The listing builds one solid part. Answer for the finished solid, in the listing's coordinates (mm). Face numbers are marked on the shaded views. A direction names the side the tool comes from. Coordinates: 2 decimals unless noted, no trailing zeros. Loops run counter-clockwise (first coordinate to the right, second up) from the corner with the lowest first, then second, coordinate; pieces in that order, holes last. Notation, with made-up numbers: (-6, 12.5) - (14, 12.5) arc R25 ccw to (14, 24.5) - close; hole circle Ø8 at (-38.75, 32). An arc over 180 degrees is marked (long way). Put each result on its own line as item: value.
```python
from build123d import *

# Parameters (mm, degrees)
SKETCH1_W               = 120
SKETCH1_H               = 31.25
BOSS_EXTRUDE1_DEPTH     = 7
SKETCH2_W               = 120
SKETCH2_H               = 4
SKETCH2_H_2             = 1
BOSS_EXTRUDE2_DEPTH     = 8
CUT_EXTRUDE1_DEPTH      = 125.260059955
CUT_EXTRUDE1_DEPTH_BACK = 125.260059955
SKETCH3_W               = 102
SKETCH3_H               = 8
SKETCH3_H_2             = 3.5
CUT_EXTRUDE3_REACH      = 126.906
SKETCH6_W               = 5
SKETCH6_H               = 1
SKETCH4_W               = 3
SKETCH4_H               = 8.090611825
SKETCH4_H_2             = 10.659388175
CUT_EXTRUDE4_DEPTH      = 5
SKETCH5_W               = 2.75
SKETCH5_H               = 7.59
SKETCH5_H_2             = 11.2
BOSS_EXTRUDE3_DEPTH     = 5
SKETCH7_R               = 3.1
CUT_EXTRUDE5_DEPTH      = 4
CUT_EXTRUDE6_START      = -1
SKETCH8_R               = 3.1
CUT_EXTRUDE6_DEPTH      = 1
CHAMFER1_SIZE           = 1


with BuildPart() as part:
    # Sketch1 → Boss-Extrude1 (new body)
    with BuildSketch(Plane.XY):
        with Locations((60, 15.625)):
            Rectangle(SKETCH1_W, SKETCH1_H)
    extrude(amount=BOSS_EXTRUDE1_DEPTH)

    # Sketch2 → Boss-Extrude2 (add)
    with BuildSketch(Plane.XY.offset(7)):
        with Locations((60, 25.6)):
            Rectangle(SKETCH2_W, SKETCH2_H)
        with Locations((60, 0.5)):
            Rectangle(SKETCH2_W, SKETCH2_H_2)
    extrude(amount=BOSS_EXTRUDE2_DEPTH)

    # Sketch3 → Cut-Extrude1 (cut, two sides: drawn at the far end of the back side and taken through both)
    with BuildSketch(Plane.XY.offset(7).offset(-CUT_EXTRUDE1_DEPTH_BACK)):
        with Locations((61, 11.1)):
            Rectangle(SKETCH3_W, SKETCH3_H)
        with Locations((61, 21.85)):
            Rectangle(SKETCH3_W, SKETCH3_H_2)
    extrude(amount=CUT_EXTRUDE1_DEPTH + CUT_EXTRUDE1_DEPTH_BACK, mode=Mode.SUBTRACT)

    # Sketch6 → Cut-Extrude3 (cut, up to next)
    with BuildSketch(Plane.ZY, mode=Mode.PRIVATE) as cut_extrude3_sk1:
        with Locations((12.5, 0.5)):
            Rectangle(SKETCH6_W, SKETCH6_H)
    cut_extrude3_tool1 = extrude(cut_extrude3_sk1.sketch, amount=-CUT_EXTRUDE3_REACH, mode=Mode.PRIVATE) & part.part
    add(cut_extrude3_tool1.solids().sort_by_distance((0, 0.5, 12.5))[0], mode=Mode.SUBTRACT)

    # Sketch4 → Cut-Extrude4 (cut)
    with BuildSketch(Plane.ZY):
        with Locations((3.5, 24.204694088)):
            Rectangle(SKETCH4_W, SKETCH4_H)
        with Locations((3.5, 8.829694088)):
            Rectangle(SKETCH4_W, SKETCH4_H_2)
    extrude(amount=-CUT_EXTRUDE4_DEPTH, mode=Mode.SUBTRACT)

    # Sketch5 → Boss-Extrude3 (add)
    with BuildSketch(Plane(origin=(120, 0, 0), x_dir=(0, 0, -1), z_dir=(1, 0, 0))):
        with Locations((-3.5, 24.205)):
            Rectangle(SKETCH5_W, SKETCH5_H)
        with Locations((-3.5, 9.35)):
            Rectangle(SKETCH5_W, SKETCH5_H_2)
    extrude(amount=BOSS_EXTRUDE3_DEPTH)

    # Sketch7 → Cut-Extrude5 (cut)
    with BuildSketch(Plane.XY.offset(7)):
        with Locations((116, 15.1)):
            Circle(SKETCH7_R)
    extrude(amount=-CUT_EXTRUDE5_DEPTH, mode=Mode.SUBTRACT)

    # Sketch8 → Cut-Extrude6 (cut)
    with BuildSketch(Plane(origin=(0, 0, 0), x_dir=(-1, 0, 0), z_dir=(0, 0, -1)).offset(CUT_EXTRUDE6_START)):
        with Locations(Location((-116, 15.1, 0), (0, 0, 180))):
            Circle(SKETCH8_R)
    extrude(amount=CUT_EXTRUDE6_DEPTH, mode=Mode.SUBTRACT)

    # Chamfer1
    chamfer1_edges = [part.edges().sort_by_distance(p)[0] for p in [
        (112.9, 15.1, 1),
    ]]
    chamfer(chamfer1_edges, length=CHAMFER1_SIZE - 0.0001)  # a hair under: the kernel refuses the full size


solid = part.part
```
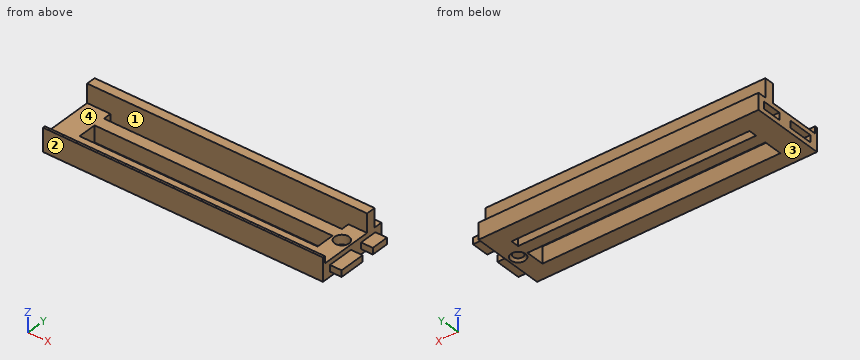
1) The part is cut by section B-B (z = 8.25). Give the vertices of the cut face in (x, y), and give its area (3 significant figures).
Found:
outline: (0, 0) - (120, 0) - (120, 1) - (0, 1) - close; (0, 23.6) - (120, 23.6) - (120, 27.6) - (0, 27.6) - close
area: 600 mm^2
2) Each of these flat-tipped pins is pushed along its axis until it touches: pin 1 (11.5 mm diameter, centred on x = 70, y = 8, fed in from +Z); pin 2 (3 mm diameter, centred on x = 38.5, y = 13, fed in from -Z); pin 3 (0.8 mm diameter, centred on x = 40.5, y = 0.5, fed in from +Z); pin 4 (1.4 mm diameter, centred on x = 123, z = 3, fed in from +Y). Where does it stop, or does it pass through?
Found:
pin 1: stops at z = 7
pin 2: passes through
pin 3: stops at z = 10
pin 4: stops at y = 28
3) The part is cut by section D-D (y = 5). Give the vertices of the cut face in (x, z) (3 decimals).
Found:
outline: (0, 0) - (120, 0) - (120, 2.125) - (125, 2.125) - (125, 4.875) - (120, 4.875) - (120, 7) - (0, 7) - (0, 5) - (5, 5) - (5, 2) - (0, 2) - close
4) For a pull along X with two mould halves and no side action, classify the marked faces 1 and 2 as pulls with the +X half, pulls with the -X half, needs draft (parallel to the pull), parting line crosses it, or undercut.
Found:
face 1: undercut
face 2: needs draft
5) For the marked faces 3 and 4, determine the directions among +Z, -Z, +X, -X, +Y, -Y from which every point of the face is accessible in a straight line to the end or side of a thin tool.
Found:
face 3: -Z, +X, -X, +Y, -Y
face 4: +Z, +X, -X
6) Straight lines are drawn through the part: L1, parallel to Y at x = 97.5, z = 4.75; L2, parallel to Y at x = 61.5, z = 9.25; L3, parallel to Y at x = 53, z = 14.75. For each, find the intervals that lie inside material, in ascending order. Write a range as [from, to].
Found:
L1: y = [0, 7.1], [15.1, 20.1], [23.6, 31.25]
L2: y = [0, 1], [23.6, 27.6]
L3: y = [23.6, 27.6]
7) The part is cut by section A-A (x = 31.5). Give the vertices of the cut face in (y, z), and give its area (3 significant figures).
Found:
outline: (0, 0) - (7.1, 0) - (7.1, 7) - (1, 7) - (1, 10) - (0, 10) - close; (15.1, 0) - (20.1, 0) - (20.1, 7) - (15.1, 7) - close; (23.6, 0) - (31.25, 0) - (31.25, 7) - (27.6, 7) - (27.6, 15) - (23.6, 15) - close
area: 173 mm^2
